For this review, take the finished solid that the model builds, in its own axes (mm). A direction names the side the tool comes from. Coordinates: 2 decimals unless noted, no trailing zeros. Loops run counter-clockwise (first coordinate to the right, second up) from the corner with the lowest first, then second, coordinate; pieces in that order, holes last. Notation, with made-up numbers: M -23,-39.75 L 18,-39.75 A26 cw 18,-10.75 Z; hole C -24,-2.75 d7. An arc over 180 degrees is marked long. Use one line per item in the form item = value.
```python
from build123d import *

# Parameters (mm, degrees)
BOSS_EXTRUDE1_DEPTH = 4.5
CUT_EXTRUDE1_DEPTH  = 4
SKETCH3_W           = 13.5
SKETCH3_H           = 6
CUT_EXTRUDE2_DEPTH  = 15


with BuildPart() as part:
    # Sketch1 → Boss-Extrude1 (new body)
    with BuildSketch(Plane(origin=(0, 0, 0), x_dir=(1, 0, 0), z_dir=(0, 1, 0))):
        with BuildLine():
            Line((-21.75, -32.5), (21.75, -32.5))
            ThreePointArc((21.75, -32.5), (24.224873734, -31.474873734), (25.25, -29))
            Line((25.25, -29), (25.25, 29))
            ThreePointArc((25.25, 29), (24.224873734, 31.474873734), (21.75, 32.5))
            Line((21.75, 32.5), (-21.75, 32.5))
            ThreePointArc((-21.75, 32.5), (-24.224873734, 31.474873734), (-25.25, 29))
            Line((-25.25, 29), (-25.25, -29))
            ThreePointArc((-25.25, -29), (-24.224873734, -31.474873734), (-21.75, -32.5))
        make_face()
    extrude(amount=BOSS_EXTRUDE1_DEPTH)

    # Sketch2 → Cut-Extrude1 (cut)
    with BuildSketch(Plane.XZ):
        with BuildLine():
            Line((-19.75, -30.5), (19.75, -30.5))
            ThreePointArc((19.75, -30.5), (22.224873734, -29.474873734), (23.25, -27))
            Line((23.25, -27), (23.25, 27))
            ThreePointArc((23.25, 27), (22.224873734, 29.474873734), (19.75, 30.5))
            Line((19.75, 30.5), (-19.75, 30.5))
            ThreePointArc((-19.75, 30.5), (-22.224873734, 29.474873734), (-23.25, 27))
            Line((-23.25, 27), (-23.25, -27))
            ThreePointArc((-23.25, -27), (-22.224873734, -29.474873734), (-19.75, -30.5))
        make_face()
    extrude(amount=-CUT_EXTRUDE1_DEPTH, mode=Mode.SUBTRACT)

    # Sketch3 → Cut-Extrude2 (cut)
    with BuildSketch(Plane.XY.offset(32.5)):
        Rectangle(SKETCH3_W, SKETCH3_H)
    extrude(amount=-CUT_EXTRUDE2_DEPTH, mode=Mode.SUBTRACT)


solid = part.part
```
1. Consider section B-B on x = 4. Write out the cut boundary in (y, z), plus the area to 3 significant figures.
Computed values:
outline = M 0,-32.5 L 4.5,-32.5 L 4.5,32.5 L 3,32.5 L 3,30.5 L 4,30.5 L 4,-30.5 L 0,-30.5 Z
area = 42.5 mm2
2. Wall thickness on line 1 along X through (y, z) = (2.75, -0.5); line 2 along Z through (x, y) = (-9.5, 0.75); line 3 along Z through (x, y) = (-2, 1.65): over which ranges is each line inside the solid? List them lowest first. Write a range as from..to.
Computed values:
line_1 = -25.25..-23.25, 23.25..25.25
line_2 = -32.5..-30.5, 30.5..32.5
line_3 = -32.5..-30.5
3. Tool access review of faces 4 (the face through (-6.75, 1, 32)), 5 (the face through (-24.3, 2.2, 31.4)), 6 (the face through (0, 4, 0)): name each direction out of +Z, -Z, +X, -X, +Y, -Y from which nothing blocks a thin tool from reaching the whole face with its end or side.
Computed values:
face_4 = +Z, -Y
face_5 = +Z, -X, +Y, -Y
face_6 = -Y
4. Draft analysis for pull direction Z (two halves, no side actions). For faces 1 (the face through (24.3, 2.2, -31.4)), 2 (the face through (24, 0, -3)), 3 (the face through (0.3, 3.3, 30.5)), state which applies: +Z half, -Z half, draft (parallel to the pull), parting line (faces both ways), or undercut.
Computed values:
face_1 = -Z half
face_2 = draft
face_3 = undercut
5. For pin 1 Ø2 at (x, y) = (-0.5, 1.5) entering from +Z; pin 2 Ø0.6 at (y, z) = (1, 32) entering from -X; pin 3 Ø0.6 at (x, z) = (0.5, 31.5) entering from -Y, all flat-tipped, find the tip position at first contact; note any pin that passes through.
Computed values:
pin_1 = -30.5
pin_2 = -23.98
pin_3 = 3
6. Consider section A-A on z = -23. Write out the cut boundary in (x, y), plus the area to 4 significant figures.
Computed values:
outline = M -25.25,0 L -23.25,0 L -23.25,4 L 23.25,4 L 23.25,0 L 25.25,0 L 25.25,4.5 L -25.25,4.5 Z
area = 41.25 mm2
7. Consider section C-C on y = 1.2. Write out the cut boundary in (x, z), plus the area to 3 significant figures.
Computed values:
outline = M -25.25,-29 A3.5 ccw -21.75,-32.5 L 21.75,-32.5 A3.5 ccw 25.25,-29 L 25.25,29 A3.5 ccw 21.75,32.5 L 6.75,32.5 L 6.75,30.5 L 19.75,30.5 A3.5 cw 23.25,27 L 23.25,-27 A3.5 cw 19.75,-30.5 L -19.75,-30.5 A3.5 cw -23.25,-27 L -23.25,27 A3.5 cw -19.75,30.5 L -6.75,30.5 L -6.75,32.5 L -21.75,32.5 A3.5 ccw -25.25,29 Z
area = 419 mm2
